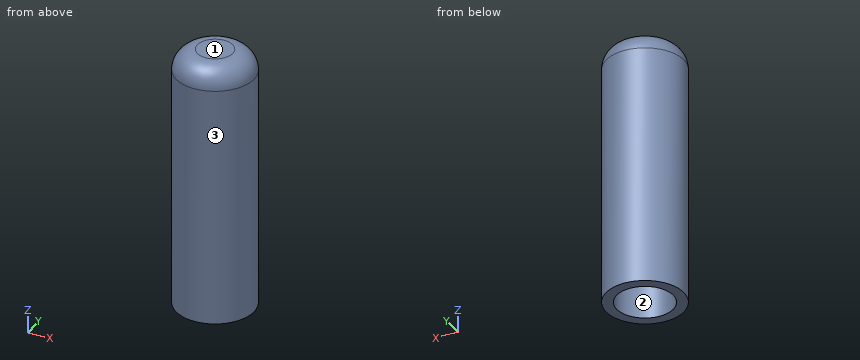
```python
from build123d import *

# Parameters (mm, degrees)
F0_R     = 5.5
F1_DEPTH = 25
F2_R     = 4
F3_DEPTH = 10
F4_R     = 3
F5_DEPTH = 12


with BuildPart() as f1:
    # F0 (on Top) → F1 (new body)
    with BuildSketch(Plane.XY):
        Circle(F0_R)
    extrude(amount=F1_DEPTH)

    # F2 (on face) → F3 (cut)
    with BuildSketch(Plane(origin=(0, 0, 0), x_dir=(1, 0, 0), z_dir=(0, 0, -1))):
        Circle(F2_R)
    extrude(amount=-F3_DEPTH, mode=Mode.SUBTRACT)

    # F4
    f4_edges = [f1.edges().sort_by_distance(p)[0] for p in [
        (-5.5, 0, 25),
    ]]
    fillet(f4_edges, radius=F4_R)

    # F5 (add): a face of the model
    f5_faces = [f1.faces().sort_by_distance(p)[0] for p in [
        (-5.3444365081, 0, 0),
    ]]
    extrude(f5_faces, amount=F5_DEPTH)


solid = f1.part
```
Can you work these out from the model? Positions are in its coordinate system, mm. Face numbers are marked on the shaded views. Coordinates: 2 decimals unless noted, no trailing zeros. Order: outer loops, then holes, each group sorted by start corner. A loop starts at its lowest first (then second) coordinate and runs counter-clockwise, first axis right, second up.
1. I need wall thicknesses on line 1 (Y direction, x = 0, z = -7.25); line 2 (Z direction, x = -0.25, y = -1.5); line 3 (Y direction, x = 3, z = -9). Which ranges of each line are inside material? Lowest first, please.
2. If we section it at B-B (z = 17): Please give me the cut outline in (x, y), then the cut area to 3 significant figures.
3. Thinking about a two-plate mould opening in X: for the marked faces 1, 2 and 3, which applies, +X half, -X half, draft (parallel to the pull), parting line (faces both ways), or undercut?
4. If we section it at A-A (z = -1): Please give me the cut outline in (x, y), then the cut area to 3 significant figures.
5. I'm going to push flat-ended pins straight in: pin 1 (1.5 mm diameter, centred on y = -2.5, z = 15.5, fed in from +X); pin 2 (6 mm diameter, centred on y = -4, z = 1.5, fed in from -X). Where does each tip first touch, or does it pass through?
Entries:
1. line 1: y = -5.5 to -4, 4 to 5.5
1. line 2: z = 10 to 25
1. line 3: y = -4.61 to -2.65, 2.65 to 4.61
2. outline: circle Ø11 at (0, 0)
2. area: 95.0 mm2
3. face 1: draft
3. face 2: undercut
3. face 3: parting line
4. outline: circle Ø11 at (0, 0); hole circle Ø8 at (0, 0)
4. area: 44.8 mm2
5. pin 1: stops at x = 5.21
5. pin 2: stops at x = -5.41
